The model under review builds one solid part; all positions refer to its coordinate system, in mm. A direction names the side the tool comes from. Round coordinates to 2 decimals unless told otherwise and drop trailing zeros. Order: outer loops, then holes, each group sorted by start corner. A loop starts at its lowest first (then second) coordinate and runs counter-clockwise, first axis right, second up. Notation, with made-up numbers: M 54.5,9 L 64.5,9 A8 ccw 64.5,15 Z; hole C 11,27.25 d9. An arc over 180 degrees is marked long. Answer as a JSON object with one key per item and string values. Group by question number.
1. Add section B-B on y = 144. State the section outline as (x, z) points (1 decimal).
2. Mouldability with a two-part tool opening along Z and no side actions: class faces 1 (the face through (67.49, 147.65, -24.3)), 2 (the face through (118, 131.804, 0)), 3 (the face through (154.38, 147.39, 24.9)), 4 (the face through (110, 162.913, 12)) as released by +Z, released by -Z, zero draft, split by the parting line, or undercut.
3. Machinability: for faces 5 (the face through (56.12, 140.057, -2.204)), 6 (the face through (107.765, 123.11, -30.108)), which of the approach directions +Z, -Z, +X, -X, +Y, -Y give a long, thin tool a straight path to every point of the face, cutting with its end or side? Answer none if there is none.
4. Clearance check with flat-ended pins moving along their axes: P1, Ø1.5, axis at y = 142, z = 13, coming from the -X side; P2, Ø3, axis at x = 96.5, y = 157.5, coming from the +Z side; P3, Ø3, axis at y = 145, z = -35, coming from the +X side. State where each tip first meets the part, or that it passes through.
5. Add section C-C on z = 42.5. State the section outline as (x, y) points, and give its area (3 significant figures).
6. Add section D-D on y = 153. State the section outline as (x, z) points (1 decimal).
7. To check wall thickness, follow probe 1 along Y at (x, z) = (128.5, 14); probe 2 along X at (y, z) = (132.5, -1.5); probe 3 along X at (y, z) = (142.5, 0). State the ranges of each line that lie inside material, in increasing order. Write a range as [from, to].
```python
from build123d import *

# Parameters (mm, degrees)
BOSS_EXTRUDE1_DEPTH = 50.8
CUT_EXTRUDE1_REACH  = 267.827
SKETCH3_W           = 270.689015678
SKETCH3_H           = 127.641974873
SKETCH4_W           = 182.593572116
SKETCH4_H           = 90.656556142
CUT_EXTRUDE2_DEPTH  = 276.287495976
SKETCH5_R           = 4.7625
CUT_EXTRUDE3_DEPTH  = 234.611541089


# Read off the part's stored shape, not the designer's step: Cavity1
with BuildPart() as part:
    # Sketch1 → Boss-Extrude1 (new body)
    with BuildSketch(Plane.XY):
        Polygon((0, 162.912922238), (223.435555158, 162.912922238), (111.717777579, 117.412759364), align=None)
    boss_extrude1 = extrude(amount=BOSS_EXTRUDE1_DEPTH)

    # Sketch3 → Cut-Extrude1 (cut, up to next)
    with BuildSketch(Plane(origin=(22.441501566, 20.662959115, -49.352651191), x_dir=(0.9221668342969159, -0.1493780822790374, 0.35678357341312894), z_dir=(-0.38679235995919625, -0.3561381441534573, 0.8506217094314763)), mode=Mode.PRIVATE) as cut_extrude1_sk1:
        with Locations((94.443721281, 144.982742911)):
            Rectangle(SKETCH3_W, SKETCH3_H)
    cut_extrude1_tool1 = extrude(cut_extrude1_sk1.sketch, amount=CUT_EXTRUDE1_REACH, mode=Mode.PRIVATE) & part.part
    cut_extrude1 = cut_extrude1_tool1.solids().sort_by_distance((109.534369, 140.289581, 40.33523))[0]
    add(cut_extrude1, mode=Mode.SUBTRACT)

    # Sketch4 → Cut-Extrude2 (cut, through all)
    with BuildSketch(Plane(origin=(10.986318642, -10.115626722, 24.160769733), x_dir=(0.9221668342969159, 0.14937808227903746, -0.35678357341312883), z_dir=(0.3867923599591962, -0.3561381441534575, 0.8506217094314763))):
        with Locations((161.909836557, 133.814028117)):
            Rectangle(SKETCH4_W, SKETCH4_H)
    cut_extrude2 = extrude(amount=CUT_EXTRUDE2_DEPTH, mode=Mode.SUBTRACT)

    # Mirror1: Boss-Extrude1, Cut-Extrude1, Cut-Extrude2 across plane
    add(boss_extrude1.mirror(Plane.XY))
    add(cut_extrude1.mirror(Plane.XY), mode=Mode.SUBTRACT)
    add(cut_extrude2.mirror(Plane.XY), mode=Mode.SUBTRACT)

    # Sketch5 → Cut-Extrude3 (cut, through all)
    with BuildSketch(Plane(origin=(0, 162.912922238, 0), x_dir=(1, 0, 0), z_dir=(0, 1, 0))):
        with Locations(Location((111.717777579, 0, 0), (0, 0, 270))):
            Circle(SKETCH5_R)
    extrude(amount=-CUT_EXTRUDE3_DEPTH, mode=Mode.SUBTRACT)

    # Cavity1 outline → Cavity1 (revolve, cut)
    with BuildSketch(Plane(origin=(111.717777579, 0, 0), x_dir=(1, 0, 0), z_dir=(0, 0, 1))):
        Polygon((31.902660281, 131.804308366), (4.7625, 131.804308366), (4.7625, 117.412759364), (29.360304621, 117.412759364), align=None)
    revolve(axis=Axis((111.717777579, 0, 0), (0, 1, 0)), mode=Mode.SUBTRACT)


solid = part.part
```
Recorded:
{
 "1": {"outline": "M 46.4,-13.2 L 111.7,-42.9 L 177,-13.2 L 177,13.2 L 111.7,42.9 L 46.4,13.2 Z; hole C 111.7,0 d9.5"},
 "2": {"face 1": "released by -Z", "face 2": "undercut", "face 3": "released by +Z", "face 4": "zero draft"},
 "3": {"face 5": "+Z, -Z, -X, -Y", "face 6": "none"},
 "4": {"P1": "stops at x = 49.51", "P2": "stops at z = 42.54", "P3": "stops at x = 133.55"},
 "5": {"outline": "M 93.46,162.91 L 111.72,143.09 L 129.97,162.91 Z", "area": "362 mm²"},
 "6": {"outline": "M 24.3,-6.9 L 111.7,-46.6 L 199.1,-6.9 L 199.1,6.9 L 111.7,46.6 L 24.3,6.9 Z; hole C 111.7,0 d9.5"},
 "7": {"probe 1": "y = [131.8, 162.91]", "probe 2": "x = [74.67, 107.2], [116.24, 148.76]", "probe 3": "x = [50.12, 106.96], [116.48, 173.32]"}
}
